from build123d import *

# Parameters (mm, degrees)
BOSS_EXTRUDE1_DEPTH = 5
FILLET1_R           = 5
CUT_EXTRUDE1_REACH  = 7
SKETCH2_W           = 5
SKETCH2_H           = 4
CUT_EXTRUDE2_REACH  = 7
SKETCH3_R           = 1.5


with BuildPart() as part:
    # Sketch1 → Boss-Extrude1 (new body)
    with BuildSketch(Plane(origin=(0, 0, 0), x_dir=(0, 0, -1), z_dir=(1, 0, 0))):
        Polygon((-59.36916415, -47.818646587), (0, -47.818646587), (59.36916415, -47.818646587), (59.36916415, -41), (55.86916415, -41), (55.86916415, 41), (59.36916415, 41), (59.36916415, 47.818646587), (-59.36916415, 47.818646587), (-59.36916415, 41), (-55.86916415, 41), (-55.86916415, -41), (-59.36916415, -41), align=None)
        Polygon((21.702610628, -39.175443067), (21.702610628, -34.307045578), (23.024909313, -32.569779859), (30.179141539, -32.569779859), (30.179141539, -42.076978078), (35.179141539, -42.076978078), (35.179141539, -29.710380013), (48.63820865, -29.710380013), (48.63820865, 19.945173818), (35.179141539, 19.945173818), (35.179141539, 42.076978078), (30.179141539, 42.076978078), (30.179141539, 32.288188968), (23.024909313, 32.288188968), (21.287643594, 33.610487654), (21.287643594, 39.175443067), (-48.63820865, 39.175443067), (-48.63820865, -39.175443067), align=None, mode=Mode.SUBTRACT)
    extrude(amount=BOSS_EXTRUDE1_DEPTH)

    # Fillet1
    fillet1_edges = [part.edges().sort_by_distance(p)[0] for p in [
        (2.5, -47.818646587, -59.36916415),
        (2.5, -47.818646587, 59.36916415),
        (2.5, 47.818646587, 59.36916415),
        (2.5, 47.818646587, -59.36916415),
    ]]
    fillet(fillet1_edges, radius=FILLET1_R)

    # Sketch2 → Cut-Extrude1 (cut, up to next)
    with BuildSketch(Plane.ZY, mode=Mode.PRIVATE) as cut_extrude1_sk1:
        with Locations((46.13820865, 41.175443067)):
            Rectangle(SKETCH2_W, SKETCH2_H)
    cut_extrude1_tool1 = extrude(cut_extrude1_sk1.sketch, amount=-CUT_EXTRUDE1_REACH, mode=Mode.PRIVATE) & part.part
    add(cut_extrude1_tool1.solids().sort_by_distance((0, 41.175443, 46.138209))[0], mode=Mode.SUBTRACT)
    # Sketch2 → Cut-Extrude1 (cut, up to next)
    with BuildSketch(Plane.ZY, mode=Mode.PRIVATE) as cut_extrude1_sk2:
        with Locations((46.13820865, -41.175443067)):
            Rectangle(SKETCH2_W, SKETCH2_H)
    cut_extrude1_tool2 = extrude(cut_extrude1_sk2.sketch, amount=-CUT_EXTRUDE1_REACH, mode=Mode.PRIVATE) & part.part
    add(cut_extrude1_tool2.solids().sort_by_distance((0, -41.175443, 46.138209))[0], mode=Mode.SUBTRACT)
    # Sketch2 → Cut-Extrude1 (cut, up to next)
    with BuildSketch(Plane.ZY, mode=Mode.PRIVATE) as cut_extrude1_sk3:
        with Locations((-0.884341096, -41.175443067)):
            Rectangle(SKETCH2_W, SKETCH2_H)
    cut_extrude1_tool3 = extrude(cut_extrude1_sk3.sketch, amount=-CUT_EXTRUDE1_REACH, mode=Mode.PRIVATE) & part.part
    add(cut_extrude1_tool3.solids().sort_by_distance((0, -41.175443, -0.884341))[0], mode=Mode.SUBTRACT)
    # Sketch2 → Cut-Extrude1 (cut, up to next)
    with BuildSketch(Plane.ZY, mode=Mode.PRIVATE) as cut_extrude1_sk4:
        with Locations((-0.884341096, 41.175443067)):
            Rectangle(SKETCH2_W, SKETCH2_H)
    cut_extrude1_tool4 = extrude(cut_extrude1_sk4.sketch, amount=-CUT_EXTRUDE1_REACH, mode=Mode.PRIVATE) & part.part
    add(cut_extrude1_tool4.solids().sort_by_distance((0, 41.175443, -0.884341))[0], mode=Mode.SUBTRACT)

    # Sketch3 → Cut-Extrude2 (cut, up to next)
    with BuildSketch(Plane.ZY, mode=Mode.PRIVATE) as cut_extrude2_sk1:
        with Locations((-35.179141539, 42.076978078)):
            Circle(SKETCH3_R)
    cut_extrude2_tool1 = extrude(cut_extrude2_sk1.sketch, amount=-CUT_EXTRUDE2_REACH, mode=Mode.PRIVATE) & part.part
    add(cut_extrude2_tool1.solids().sort_by_distance((0, 42.076978, -35.179142))[0], mode=Mode.SUBTRACT)
    # Sketch3 → Cut-Extrude2 (cut, up to next)
    with BuildSketch(Plane.ZY, mode=Mode.PRIVATE) as cut_extrude2_sk2:
        with Locations((-30.179141539, 42.076978078)):
            Circle(SKETCH3_R)
    cut_extrude2_tool2 = extrude(cut_extrude2_sk2.sketch, amount=-CUT_EXTRUDE2_REACH, mode=Mode.PRIVATE) & part.part
    add(cut_extrude2_tool2.solids().sort_by_distance((0, 42.076978, -30.179142))[0], mode=Mode.SUBTRACT)
    # Sketch3 → Cut-Extrude2 (cut, up to next)
    with BuildSketch(Plane.ZY, mode=Mode.PRIVATE) as cut_extrude2_sk3:
        with Locations((-3.384341096, 43.175443067)):
            Circle(SKETCH3_R)
    cut_extrude2_tool3 = extrude(cut_extrude2_sk3.sketch, amount=-CUT_EXTRUDE2_REACH, mode=Mode.PRIVATE) & part.part
    add(cut_extrude2_tool3.solids().sort_by_distance((0, 43.175443, -3.384341))[0], mode=Mode.SUBTRACT)
    # Sketch3 → Cut-Extrude2 (cut, up to next)
    with BuildSketch(Plane.ZY, mode=Mode.PRIVATE) as cut_extrude2_sk4:
        with Locations((1.615658904, 43.175443067)):
            Circle(SKETCH3_R)
    cut_extrude2_tool4 = extrude(cut_extrude2_sk4.sketch, amount=-CUT_EXTRUDE2_REACH, mode=Mode.PRIVATE) & part.part
    add(cut_extrude2_tool4.solids().sort_by_distance((0, 43.175443, 1.615659))[0], mode=Mode.SUBTRACT)
    # Sketch3 → Cut-Extrude2 (cut, up to next)
    with BuildSketch(Plane.ZY, mode=Mode.PRIVATE) as cut_extrude2_sk5:
        with Locations((-55.86916415, 41)):
            Circle(SKETCH3_R)
    cut_extrude2_tool5 = extrude(cut_extrude2_sk5.sketch, amount=-CUT_EXTRUDE2_REACH, mode=Mode.PRIVATE) & part.part
    add(cut_extrude2_tool5.solids().sort_by_distance((0, 41, -55.869164))[0], mode=Mode.SUBTRACT)
    # Sketch3 → Cut-Extrude2 (cut, up to next)
    with BuildSketch(Plane.ZY, mode=Mode.PRIVATE) as cut_extrude2_sk6:
        with Locations((43.63820865, 43.175443067)):
            Circle(SKETCH3_R)
    cut_extrude2_tool6 = extrude(cut_extrude2_sk6.sketch, amount=-CUT_EXTRUDE2_REACH, mode=Mode.PRIVATE) & part.part
    add(cut_extrude2_tool6.solids().sort_by_distance((0, 43.175443, 43.638209))[0], mode=Mode.SUBTRACT)
    # Sketch3 → Cut-Extrude2 (cut, up to next)
    with BuildSketch(Plane.ZY, mode=Mode.PRIVATE) as cut_extrude2_sk7:
        with Locations((48.63820865, 43.175443067)):
            Circle(SKETCH3_R)
    cut_extrude2_tool7 = extrude(cut_extrude2_sk7.sketch, amount=-CUT_EXTRUDE2_REACH, mode=Mode.PRIVATE) & part.part
    add(cut_extrude2_tool7.solids().sort_by_distance((0, 43.175443, 48.638209))[0], mode=Mode.SUBTRACT)
    # Sketch3 → Cut-Extrude2 (cut, up to next)
    with BuildSketch(Plane.ZY, mode=Mode.PRIVATE) as cut_extrude2_sk8:
        with Locations((48.63820865, -43.175443067)):
            Circle(SKETCH3_R)
    cut_extrude2_tool8 = extrude(cut_extrude2_sk8.sketch, amount=-CUT_EXTRUDE2_REACH, mode=Mode.PRIVATE) & part.part
    add(cut_extrude2_tool8.solids().sort_by_distance((0, -43.175443, 48.638209))[0], mode=Mode.SUBTRACT)
    # Sketch3 → Cut-Extrude2 (cut, up to next)
    with BuildSketch(Plane.ZY, mode=Mode.PRIVATE) as cut_extrude2_sk9:
        with Locations((43.63820865, -43.175443067)):
            Circle(SKETCH3_R)
    cut_extrude2_tool9 = extrude(cut_extrude2_sk9.sketch, amount=-CUT_EXTRUDE2_REACH, mode=Mode.PRIVATE) & part.part
    add(cut_extrude2_tool9.solids().sort_by_distance((0, -43.175443, 43.638209))[0], mode=Mode.SUBTRACT)
    # Sketch3 → Cut-Extrude2 (cut, up to next)
    with BuildSketch(Plane.ZY, mode=Mode.PRIVATE) as cut_extrude2_sk10:
        with Locations((1.615658904, -43.175443067)):
            Circle(SKETCH3_R)
    cut_extrude2_tool10 = extrude(cut_extrude2_sk10.sketch, amount=-CUT_EXTRUDE2_REACH, mode=Mode.PRIVATE) & part.part
    add(cut_extrude2_tool10.solids().sort_by_distance((0, -43.175443, 1.615659))[0], mode=Mode.SUBTRACT)
    # Sketch3 → Cut-Extrude2 (cut, up to next)
    with BuildSketch(Plane.ZY, mode=Mode.PRIVATE) as cut_extrude2_sk11:
        with Locations((-3.384341096, -43.175443067)):
            Circle(SKETCH3_R)
    cut_extrude2_tool11 = extrude(cut_extrude2_sk11.sketch, amount=-CUT_EXTRUDE2_REACH, mode=Mode.PRIVATE) & part.part
    add(cut_extrude2_tool11.solids().sort_by_distance((0, -43.175443, -3.384341))[0], mode=Mode.SUBTRACT)
    # Sketch3 → Cut-Extrude2 (cut, up to next)
    with BuildSketch(Plane.ZY, mode=Mode.PRIVATE) as cut_extrude2_sk12:
        with Locations((-30.179141539, -42.076978078)):
            Circle(SKETCH3_R)
    cut_extrude2_tool12 = extrude(cut_extrude2_sk12.sketch, amount=-CUT_EXTRUDE2_REACH, mode=Mode.PRIVATE) & part.part
    add(cut_extrude2_tool12.solids().sort_by_distance((0, -42.076978, -30.179142))[0], mode=Mode.SUBTRACT)
    # Sketch3 → Cut-Extrude2 (cut, up to next)
    with BuildSketch(Plane.ZY, mode=Mode.PRIVATE) as cut_extrude2_sk13:
        with Locations((-35.179141539, -42.076978078)):
            Circle(SKETCH3_R)
    cut_extrude2_tool13 = extrude(cut_extrude2_sk13.sketch, amount=-CUT_EXTRUDE2_REACH, mode=Mode.PRIVATE) & part.part
    add(cut_extrude2_tool13.solids().sort_by_distance((0, -42.076978, -35.179142))[0], mode=Mode.SUBTRACT)
    # Sketch3 → Cut-Extrude2 (cut, up to next)
    with BuildSketch(Plane.ZY, mode=Mode.PRIVATE) as cut_extrude2_sk14:
        with Locations((-55.86916415, -41)):
            Circle(SKETCH3_R)
    cut_extrude2_tool14 = extrude(cut_extrude2_sk14.sketch, amount=-CUT_EXTRUDE2_REACH, mode=Mode.PRIVATE) & part.part
    add(cut_extrude2_tool14.solids().sort_by_distance((0, -41, -55.869164))[0], mode=Mode.SUBTRACT)
    # Sketch3 → Cut-Extrude2 (cut, up to next)
    with BuildSketch(Plane.ZY, mode=Mode.PRIVATE) as cut_extrude2_sk15:
        with Locations((55.86916415, -41)):
            Circle(SKETCH3_R)
    cut_extrude2_tool15 = extrude(cut_extrude2_sk15.sketch, amount=-CUT_EXTRUDE2_REACH, mode=Mode.PRIVATE) & part.part
    add(cut_extrude2_tool15.solids().sort_by_distance((0, -41, 55.869164))[0], mode=Mode.SUBTRACT)
    # Sketch3 → Cut-Extrude2 (cut, up to next)
    with BuildSketch(Plane.ZY, mode=Mode.PRIVATE) as cut_extrude2_sk16:
        with Locations((55.86916415, 41)):
            Circle(SKETCH3_R)
    cut_extrude2_tool16 = extrude(cut_extrude2_sk16.sketch, amount=-CUT_EXTRUDE2_REACH, mode=Mode.PRIVATE) & part.part
    add(cut_extrude2_tool16.solids().sort_by_distance((0, 41, 55.869164))[0], mode=Mode.SUBTRACT)


solid = part.part
The model under review builds one solid part; all positions refer to its coordinate system, in mm. A direction names the side the tool comes from. Coordinates: 2 decimals unless noted, no trailing zeros. Order: outer loops, then holes, each group sorted by start corner. A loop starts at its lowest first (then second) coordinate and runs counter-clockwise, first axis right, second up. Notation, with made-up numbers: (41.5, 27.5) -> (63.5, 27.5) arc R21 cw to (63.5, 48.5) -> close; hole circle Ø2 at (47, -30). An arc over 180 degrees is marked (long way). Answer in a Markdown table with one row per item.
(1) Consider section B-B (z = -10.5). Write out the cut boundary in (x, y).
Answers:
| item | result |
|---|---|
| outline | (0, -47.82) -> (5, -47.82) -> (5, -39.18) -> (0, -39.18) -> close; (0, 39.18) -> (5, 39.18) -> (5, 47.82) -> (0, 47.82) -> close |
(2) Machinability: for faces 5 (the flat face through (2, -1, -55.869)), 6 (the flat face through (2, -35, -35.179)), 7 (the flat face through (2, 1, 55.869)), which of the approach directions +Z, -Z, +X, -X, +Y, -Y give a long, thin tool a straight path to every point of the face, cutting with its end or side? Answer none if there is none.
Answers:
| item | result |
|---|---|
| face 5 | -Z, +X, -X |
| face 6 | +X, -X |
| face 7 | +Z, +X, -X |
(3) Insertion check: pin 1 (3 mm diameter, centred on x = 3.5, y = 37.5, fed in from -Z); pin 2 (1.5 mm diameter, centred on x = 3, y = -26.5, fed in from +Z); pin 3 (1.6 mm diameter, centred on x = 3, z = -58, fed in from -Y). Each pin has a flat end and moves straight along its axis. Give the tip position at first contact, or say it passes through.
Answers:
| item | result |
|---|---|
| pin 1 | z = -55.87 |
| pin 2 | z = 55.87 |
| pin 3 | y = -46.94 |
(4) The part is to be moulded in two halves that separate along Y. For faces 1 (the cylindrical face through (2.54, -46.39, 57.87)), 2 (the cylindrical face through (2.54, 46.32, -57.94)), 3 (the cylindrical face through (2.46, -44.2, 42.54)), 4 (the flat face through (2, -39.175, 23)), say which applies: +Y half, -Y half, draft (parallel to the pull), parting line (faces both ways), or undercut.
Answers:
| item | result |
|---|---|
| face 1 | -Y half |
| face 2 | +Y half |
| face 3 | undercut |
| face 4 | undercut |
(5) Consider section A-A (y = 2). Write out the cut boundary in (x, z), plus the area to 3 significant figures.
Answers:
| item | result |
|---|---|
| outline | (0, -55.87) -> (5, -55.87) -> (5, -48.64) -> (0, -48.64) -> close; (0, 48.64) -> (5, 48.64) -> (5, 55.87) -> (0, 55.87) -> close |
| area | 72.3 mm² |
(6) Wall thickness on line 1 along Z through (x, y) = (2.5, -37.5); line 2 along Z through (x, y) = (0.6, 39); line 3 along Y through (x, z) = (0.6, -17.5): over which ranges is each line inside the solid? List them lowest first.
Answers:
| item | result |
|---|---|
| line 1 | -55.87 to -35.18, -30.18 to -21.7, 48.64 to 55.87 |
| line 2 | -55.87 to -35.18, -30.18 to -21.29, 48.64 to 55.87 |
| line 3 | -47.82 to -39.18, 39.18 to 47.82 |
